The listing builds one solid part. Answer for the finished solid, in the listing's coordinates (mm). A direction names the side the tool comes from. Round coordinates to 2 decimals unless told otherwise and drop trailing zeros. Loops run counter-clockwise (first coordinate to the right, second up) from the corner with the lowest first, then second, coordinate; pieces in that order, holes last. Notation, with made-up numbers: M 45.5,-30 L 82.5,-30 A18 ccw 82.5,0 Z; hole C 63,-26.75 d5. An arc over 180 degrees is marked long. Put each result on its own line as item: value. Start each with the question number.
(1) Section A-A, the plane y = 365 is taken. Determine the outline of the cut face in (x, z).
(2) Section B-B, the plane x = 17 is taken. Determine the outline of the cut face in (y, z), then the cut area to 3 significant figures.
(3) Section C-C, the plane z = 435.5 is taken. Determine the outline of the cut face in (x, y), then the cut area to 3 significant figures.
(4) Flat-ended cylindrical pins translate along their axes: P1, Ø8, axis at y = 187.5, z = 910, coming from the -X side; P2, Ø4, axis at y = 20.5, z = 606, coming from the -X side; P3, Ø14.5, axis at x = 3, y = 356.5, coming from the -Z side; P4, Ø14.5, axis at x = 26, y = 372, coming from the +Z side. Find the tip coordinate at first contact, or state that the pin passes through.
(5) Straight lines are drawn through the part: line 1 (Z direction, x = 27, y = 273); line 2 (Y direction, x = 77, z = 257.5); line 3 (X direction, y = 25, z = 105). For each, find the intervals that lie inside material, in ascending order.
(6) Which of the six approach directions +Z, -Z, +X, -X, +Y, -Y give full straight-line access (tool end or side, diameter ignored) to faces 5 (the face through (15, 326, 803)), 6 (the face through (15, 326, 773)), 7 (the face through (10.163, 323.592, 262.35)), 8 (the face through (15, 326, 247))?
(7) Section D-D, the plane x = 89 is taken. Determine the outline of the cut face in (y, z).
(8) Determine the mould class of faces 1 (the face through (10.163, 323.592, 788.35)), 2 (the face through (65, 0, 518)), 3 (the face through (20.163, 325.356, 261.79)), 4 (the face through (103.13, 10.44, 517.65)) for opening direction X: released by +X, released by -X, zero draft, split by the parting line, or undercut.
Autodesk Inventor part; units mm, degrees
ref_plane "YZ Plane" through (0, 0, 0) normal (1, 0, 0) x (0, 1, 0)
ref_plane "XZ Plane" through (0, 0, 0) normal (0, 1, 0) x (-1, 0, 0)
ref_plane "XY Plane" through (0, 0, 0) normal (0, 0, 1) x (1, 0, 0)
sketch "Sketch1" plane through (0, 0, 0) normal (0, 0, 1) x (1, 0, 0)
  line L0 (0, 0) -> (132, 0)
  line L1 (132, 0) -> (132, 23)
  line L2 (132, 23) -> (129, 23)
  line L3 (38.7399, 220) -> (28.7399, 218.2367)
  line L4 (28.7399, 218.2367) -> (0, 0)
  line L5 (129, 23) -> (129, 15)
  line L6 (129, 15) -> (76.5186, 5.7461)
  line L7 (76.5186, 5.7461) -> (119.3723, 5.7461) construction
  line L8 (76.5186, 5.7461) -> (38.7399, 220)
  dimension "d0" = 132
  dimension "d1" = 220
  dimension "d2" = 23
  dimension "d3" = 3
  dimension "d4" = 8
  dimension "d5" = 53.291
  dimension "d6" = 10
  dimension "d7" = 90
  dimension "d8" = 10
  dimension "d9" = 10
extrude "Extrusion1" add sketch "Sketch1" along normal blind 1050
sketch "Sketch2" plane through (28.7399, 218.2367, 1050) normal (-0.1736, 0.9848, 0) x (0.9848, 0.1736, 0)
  line L0 (10.1543, 1050) -> (10.1543, 0) construction
  line L1 (0, 277) -> (10.1543, 277)
  line L2 (10.1543, 277) -> (10.1543, 247)
  line L3 (10.1543, 247) -> (0, 247)
  line L4 (0, 247) -> (0, 277)
  line L5 (0, 1050) -> (0, 0) construction
  line L6 (0, 803) -> (10.1543, 803)
  line L7 (10.1543, 803) -> (10.1543, 773)
  line L8 (10.1543, 773) -> (0, 773)
  line L9 (0, 773) -> (0, 803)
  line L10 (10.1543, 1050) -> (0, 1050) construction
  point P0 (-66.1997, 1050)
  dimension "d12" = 30
  dimension "d13" = 30
  dimension "d14" = 247
  dimension "d15" = 247
extrude "Extrusion2" add sketch "Sketch2" along normal blind 220
fillet "Fillet1" radius 3 4 edges at (0.5373, 436.6577, 788) (-9.4627, 434.8944, 788) (0.5373, 436.6577, 262) (-9.4627, 434.8944, 262)
fillet "Fillet2" radius 10 4 edges at (33.7399, 219.1184, 803) (33.7399, 219.1184, 277) (33.7399, 219.1184, 773) (33.7399, 219.1184, 247)
properties part number "sostenedor1"
Recorded:
1. outline: M 2.86,247 L 13.17,247 L 13.17,277 L 2.86,277 Z; M 2.86,773 L 13.17,773 L 13.17,803 L 2.86,803 Z
2. outline: M 0,0 L 129.09,0 L 129.09,1050 L 0,1050 Z; M 284.82,247 L 343.29,247 L 343.29,277 L 284.82,277 Z; M 284.82,773 L 343.29,773 L 343.29,803 L 284.82,803 Z
2. area: 139,000 mm²
3. outline: M 0,0 L 132,0 L 132,23 L 129,23 L 129,15 L 76.52,5.75 L 38.74,220 L 28.74,218.24 Z
3. area: 10,200 mm²
4. P1: stops at x = 24.17
4. P2: stops at x = 2.44
4. P3: stops at z = 247
4. P4: passes through
5. line 1: z = 247 to 277, 773 to 803
5. line 2: y = 0 to 5.83
5. line 3: x = 3.29 to 73.12
6. face 5: +Z, +X, -X, +Y
6. face 6: +X, -X, +Y
6. face 7: +Z, -Z, -X
6. face 8: -Z, +X, -X, +Y
7. outline: M 0,0 L 7.95,0 L 7.95,1050 L 0,1050 Z
8. face 1: released by -X
8. face 2: zero draft
8. face 3: released by +X
8. face 4: undercut
